Check sheet for the modelled part. Datum: model origin and axes. Units: mm. A direction names the side the tool comes from. Round coordinates to 2 decimals unless told otherwise and drop trailing zeros. Order: outer loops, then holes, each group sorted by start corner. A loop starts at its lowest first (then second) coordinate and runs counter-clockwise, first axis right, second up.
(1) Mould release check, pull along Y, two halves, no side actions. Record for faces 5 (the flat face through (0, 18, -20.5)), 6 (the cylindrical face through (0, 35, -12)), 7 (the flat face through (-2, 40.5, -8)): released by +Y, released by -Y, zero draft, split by the parting line, or undercut.
(2) Sectioned sample at B-B, the plane y = 26.5. Enter the section's corners in (x, z).
(3) Tool access check on faces 1 (the flat face through (0, 33, 23)), 2 (the cylindrical face through (-0.07, 37.99, 15.31)), 3 (the flat face through (0, 3.3, -21)), 4 (the flat face through (0, 24.5, -11)). Record the directions out of +Z, -Z, +X, -X, +Y, -Y that give a thin tool (end or side, any length) a straight path to the whole face; none if there is none.
(4) Depth check by flat-ended pin: pin 1 (12 mm diameter, centred on x = -6, z = 0, fed in from +Y); pin 2 (1.5 mm diameter, centred on y = 32, z = -24.5, fed in from +X); pin 3 (3.5 mm diameter, centred on x = 3, z = 23.5, fed in from +Y). Enter the tip coordinate at first touch or a pass-through.
(5) Sectioned sample at A-A, the plane z = 25.5. Enter the section's corners in (x, y) (3 decimals).
(6) Sectioned sample at D-D, the plane y = 19. Enter the section's corners in (x, z), and give its area (3 significant figures).
(7) Thickness scan on probe 1 along X at (y, z) = (32.35, -25.5) (3 decimals); probe 2 along Z at (x, y) = (-2.75, 26); probe 3 along Y at (x, z) = (-1, 21). Record the ranges inside material, lowest first.
(8) Sectioned sample at C-C, the plane z = 6.5. Enter the section's corners in (x, y).
```python
from build123d import *

# Parameters (mm, degrees)
SKETCH1_W           = 20
SKETCH1_H           = 41
BOSS_EXTRUDE1_DEPTH = 37
BOSS_EXTRUDE2_DEPTH = 2
SKETCH3_R           = 6.5
BOSS_EXTRUDE3_DEPTH = 1
SKETCH4_R           = 5.25
BOSS_EXTRUDE4_DEPTH = 0.5
SKETCH5_R           = 3
BOSS_EXTRUDE5_DEPTH = 4
SKETCH6_W           = 3.5
SKETCH6_H           = 4.5
BOSS_EXTRUDE6_DEPTH = 5.5
CUT_EXTRUDE1_DEPTH  = 5
SKETCH8_W           = 9.25
SKETCH8_H           = 3
BOSS_EXTRUDE7_DEPTH = 7
SKETCH9_W           = 18.5
SKETCH9_H           = 3
BOSS_EXTRUDE8_DEPTH = 7
FILLET1_R           = 1
SKETCH10_R          = 2.5
CUT_EXTRUDE2_DEPTH  = 7
SKETCH11_R          = 1.5
CUT_EXTRUDE3_DEPTH  = 20
FILLET2_R           = 0.25
FILLET3_R           = 2


with BuildPart() as part:
    # Sketch1 → Boss-Extrude1 (new body)
    with BuildSketch(Plane(origin=(0, 0, 0), x_dir=(1, 0, 0), z_dir=(0, 1, 0))):
        Rectangle(SKETCH1_W, SKETCH1_H)
    extrude(amount=BOSS_EXTRUDE1_DEPTH)

    # Sketch2 → Boss-Extrude2 (add)
    with BuildSketch(Plane(origin=(0, 37, 0), x_dir=(1, 0, 0), z_dir=(0, 1, 0))):
        with BuildLine():
            Line((-9, 6.141101056), (-9, -13.5))
            Line((-9, -13.5), (-4.5, -13.5))
            ThreePointArc((-4.5, -13.5), (0, -15.30958424), (4.5, -13.5))
            Line((4.5, -13.5), (9, -13.5))
            Line((9, -13.5), (9, 6.141101056))
            ThreePointArc((9, 6.141101056), (0, 20.5), (-9, 6.141101056))
        make_face()
    extrude(amount=BOSS_EXTRUDE2_DEPTH)

    # Sketch3 → Boss-Extrude3 (add)
    with BuildSketch(Plane(origin=(0, 39, 0), x_dir=(1, 0, 0), z_dir=(0, 1, 0))):
        with Locations(Location((0, 10.5, 0), (0, 0, 270))):
            Circle(SKETCH3_R)
    extrude(amount=BOSS_EXTRUDE3_DEPTH)

    # Sketch4 → Boss-Extrude4 (add)
    with BuildSketch(Plane(origin=(0, 40, 0), x_dir=(1, 0, 0), z_dir=(0, 1, 0))):
        with Locations(Location((0, 10.5, 0), (0, 0, 270))):
            Circle(SKETCH4_R)
    extrude(amount=BOSS_EXTRUDE4_DEPTH)

    # Sketch5 → Boss-Extrude5 (add)
    with BuildSketch(Plane(origin=(0, 40.5, 0), x_dir=(1, 0, 0), z_dir=(0, 1, 0))):
        with Locations(Location((0, 10.5, 0), (0, 0, 270))):
            Circle(SKETCH5_R)
    extrude(amount=BOSS_EXTRUDE5_DEPTH)

    # Sketch6 → Boss-Extrude6 (add)
    with BuildSketch(Plane(origin=(0, 0, -20.5), x_dir=(-1, 0, 0), z_dir=(0, 0, -1))):
        with Locations((-1.75, 5.25)):
            Rectangle(SKETCH6_W, SKETCH6_H)
        with Locations((1.75, 5.25)):
            Rectangle(SKETCH6_W, SKETCH6_H)
    extrude(amount=BOSS_EXTRUDE6_DEPTH)

    # Sketch7 → Cut-Extrude1 (cut)
    with BuildSketch(Plane(origin=(0, 0, -26), x_dir=(-1, 0, 0), z_dir=(0, 0, -1))):
        Polygon((3.5, 7.5), (0, 7.5), (0, 7), (2.75, 7), (2.75, 3.5), (0, 3.5), (0, 3), (3.5, 3), align=None)
        Polygon((0, 7), (0, 7.5), (-3.5, 7.5), (-3.5, 3), (0, 3), (0, 3.5), (-2.75, 3.5), (-2.75, 7), align=None)
    extrude(amount=-CUT_EXTRUDE1_DEPTH, mode=Mode.SUBTRACT)

    # Sketch8 → Boss-Extrude7 (add)
    with BuildSketch(Plane.XY.offset(20.5)):
        with Locations((4.625, 31.5)):
            Rectangle(SKETCH8_W, SKETCH8_H)
        with Locations((-4.625, 31.5)):
            Rectangle(SKETCH8_W, SKETCH8_H)
    extrude(amount=BOSS_EXTRUDE7_DEPTH)

    # Sketch9 → Boss-Extrude8 (add)
    with BuildSketch(Plane(origin=(0, 0, -20.5), x_dir=(-1, 0, 0), z_dir=(0, 0, -1))):
        with Locations((0, 31.5)):
            Rectangle(SKETCH9_W, SKETCH9_H)
    extrude(amount=BOSS_EXTRUDE8_DEPTH)

    # Fillet1
    fillet1_edges = [part.edges().sort_by_distance(p)[0] for p in [
        (-9.25, 31.5, -27.5),
        (9.25, 31.5, -27.5),
        (-9.25, 31.5, 27.5),
        (9.25, 31.5, 27.5),
    ]]
    fillet(fillet1_edges, radius=FILLET1_R)

    # Sketch10 → Cut-Extrude2 (cut)
    with BuildSketch(Plane(origin=(0, 33, 0), x_dir=(1, 0, 0), z_dir=(0, 1, 0))):
        with Locations((-4.875, 25.5)):
            Circle(SKETCH10_R)
        with Locations((4.875, 25.5)):
            Circle(SKETCH10_R)
        with Locations((4.875, -25.5)):
            Circle(SKETCH10_R)
        with Locations((-4.875, -25.5)):
            Circle(SKETCH10_R)
    extrude(amount=-CUT_EXTRUDE2_DEPTH, mode=Mode.SUBTRACT)

    # Sketch11 → Cut-Extrude3 (cut)
    with BuildSketch(Plane(origin=(0, 44.5, 0), x_dir=(1, 0, 0), z_dir=(0, 1, 0))):
        with Locations(Location((0, 10.5, 0), (0, 0, 270))):
            Circle(SKETCH11_R)
    extrude(amount=-CUT_EXTRUDE3_DEPTH, mode=Mode.SUBTRACT)

    # Fillet2
    fillet2_edges = [part.edges().sort_by_distance(p)[0] for p in [
        (-3.375, 31.5, -27.5),
        (-6.375, 31.5, -27.5),
        (6.375, 31.5, -27.5),
        (3.375, 31.5, -27.5),
        (3.375, 31.5, 27.5),
        (6.375, 31.5, 27.5),
        (-6.375, 31.5, 27.5),
        (-3.375, 31.5, 27.5),
    ]]
    fillet(fillet2_edges, radius=FILLET2_R)

    # Fillet3
    # the kernel refuses this fillet: 2 mm, written as the material it takes off along each edge
    with BuildSketch(Plane(origin=(2.75, 7, -31), x_dir=(-1, 0, 0), z_dir=(0, 0, 1))) as fillet3_piece_1:
        with BuildLine():
            CenterArc((FILLET3_R, FILLET3_R), FILLET3_R, 180, 90)
            Line((0, FILLET3_R), (0, 0))
            Line((0, 0), (FILLET3_R, 0))
        make_face()
    extrude(amount=10, mode=Mode.SUBTRACT)
    with BuildSketch(Plane(origin=(-2.75, 7, -31), x_dir=(1, 0, 0), z_dir=(0, 0, 1)), Plane(origin=(-2.75, 3.5, -31), x_dir=(0, 1, 0), z_dir=(0, 0, 1)), Plane(origin=(2.75, 3.5, -31), x_dir=(-1, 0, 0), z_dir=(0, 0, 1))) as fillet3_piece_2:
        with BuildLine():
            CenterArc((FILLET3_R, -FILLET3_R), FILLET3_R, 90, 90)
            Line((0, -FILLET3_R), (0, 0))
            Line((0, 0), (FILLET3_R, 0))
        make_face()
    extrude(amount=10, mode=Mode.SUBTRACT)


solid = part.part
```
Derived:
1. face 5: undercut
1. face 6: zero draft
1. face 7: released by +Y
2. outline: (-10, -20.5) - (10, -20.5) - (10, 20.5) - (-10, 20.5) - close; hole circle Ø3 at (0, -10.5)
3. face 1: +Z, +X, -X, +Y
3. face 2: +Z, +Y
3. face 3: -Z
3. face 4: +Y
4. pin 1: stops at y = 40
4. pin 2: stops at x = 9.25
4. pin 3: stops at y = 33
5. outline: (-9.25, 30) - (-7.375, 30) - (-7.375, 33) - (-9.25, 33) - close; (-2.375, 30) - (2.375, 30) - (2.375, 33) - (-2.375, 33) - close; (7.375, 30) - (9.25, 30) - (9.25, 33) - (7.375, 33) - close
6. outline: (-10, -20.5) - (10, -20.5) - (10, 20.5) - (-10, 20.5) - close
6. area: 820 mm2
7. probe 1: x = -9.25 to -7.375, -2.375 to 2.375, 7.375 to 9.25
7. probe 2: z = -20.5 to 20.5
7. probe 3: y = 30 to 33
8. outline: (-10, 0) - (10, 0) - (10, 37) - (9, 37) - (9, 39) - (-9, 39) - (-9, 37) - (-10, 37) - close
